Design review of the part built by this model. Coordinates are the model's own, in mm. A direction names the side the tool comes from. Coordinates: 2 decimals unless noted, no trailing zeros. Write each loop counter-clockwise with the first axis right and the second up, starting at its lowest first coordinate (ties: lowest second). Pieces come first, ordered by that corner, then holes. Notation, with made-up numbers: (-20.5, -30) - (27.5, -30) arc R31 cw to (27.5, 8) - close; hole circle Ø2 at (18, -6). An arc over 180 degrees is marked (long way). Use a Markdown table: item, result.
from build123d import *

# Parameters (mm, degrees)
F0_W     = 457.2
F0_H     = 660.4
F1_DEPTH = 12.7
F3_DEPTH = 101.6


with BuildPart() as f1:
    # F0 (on Top) → F1 (new body)
    with BuildSketch(Plane.XY):
        with Locations((-228.6, 330.2)):
            Rectangle(F0_W, F0_H)
    extrude(amount=F1_DEPTH)

    # F2 (on face) → F3 (join)
    with BuildSketch(Plane.XY.offset(12.7)):
        Polygon((0, 12.7), (0, 660.4), (-12.7, 660.4), (-12.7, 647.7), (-12.7, 12.7), align=None)
        Polygon((-12.7, 647.7), (-12.7, 660.4), (-457.2, 660.4), (-457.2, 647.7), (-444.5, 647.7), align=None)
        Polygon((0, 0), (0, 12.7), (-12.7, 12.7), (-444.5, 12.7), (-444.5, 0), align=None)
        Polygon((-444.5, 12.7), (-444.5, 647.7), (-457.2, 647.7), (-457.2, 0), (-444.5, 0), align=None)
    extrude(amount=F3_DEPTH)


solid = f1.part
(1) Draft analysis for pull direction X (two halves, no side actions). For faces 1 (the flat face through (-232, 647.7, 63)), 2 (the flat face through (-457.2, 335, 56)), 3 (the flat face through (0, 326, 56)), 4 (the flat face through (-226, 12.7, 63)), state which applies: +X half, -X half, draft (parallel to the pull), parting line (faces both ways), or undercut.
Determined:
| item | result |
|---|---|
| face 1 | undercut |
| face 2 | -X half |
| face 3 | +X half |
| face 4 | undercut |
(2) For L1, parallel to X at y = 623.5, z = 89.5; L2, parallel to Y at x = -388.5, z = 76.5; L3, parallel to Z at x = -36.5, y = 276, list the stretches that pass through material, from the lowest coordinate up. Write a range as from..to.
Determined:
| item | result |
|---|---|
| L1 | -457.2..-444.5, -12.7..0 |
| L2 | 0..12.7, 647.7..660.4 |
| L3 | 0..12.7 |
(3) Take a section at C-C on x = -390. Write out the cut boundary in (y, z), and give its area (3 significant figures).
Determined:
| item | result |
|---|---|
| outline | (0, 0) - (660.4, 0) - (660.4, 114.3) - (647.7, 114.3) - (647.7, 12.7) - (12.7, 12.7) - (12.7, 114.3) - (0, 114.3) - close |
| area | 11,000 mm2 |
(4) Take a section at B-B on y = 497. Write out the cut boundary in (x, z), and give its area (3 significant figures).
Determined:
| item | result |
|---|---|
| outline | (-457.2, 0) - (0, 0) - (0, 114.3) - (-12.7, 114.3) - (-12.7, 12.7) - (-444.5, 12.7) - (-444.5, 114.3) - (-457.2, 114.3) - close |
| area | 8,390 mm2 |
(5) Machinability: for faces 5 (the flat face through (-232, 335, 0)), 6 (the flat face through (-232, 335, 12.7)), which of the approach directions +Z, -Z, +X, -X, +Y, -Y give a long, thin tool a straight path to every point of the face, cutting with its end or side? Answer none if there is none.
Determined:
| item | result |
|---|---|
| face 5 | -Z, +X, -X, +Y, -Y |
| face 6 | +Z |
(6) Take a section at A-A on z = 44. Write out the cut boundary in (x, y), and give its area (3 significant figures).
Determined:
| item | result |
|---|---|
| outline | (-457.2, 0) - (0, 0) - (0, 660.4) - (-457.2, 660.4) - close; hole (-444.5, 12.7) - (-12.7, 12.7) - (-12.7, 647.7) - (-444.5, 647.7) - close |
| area | 27,700 mm2 |
